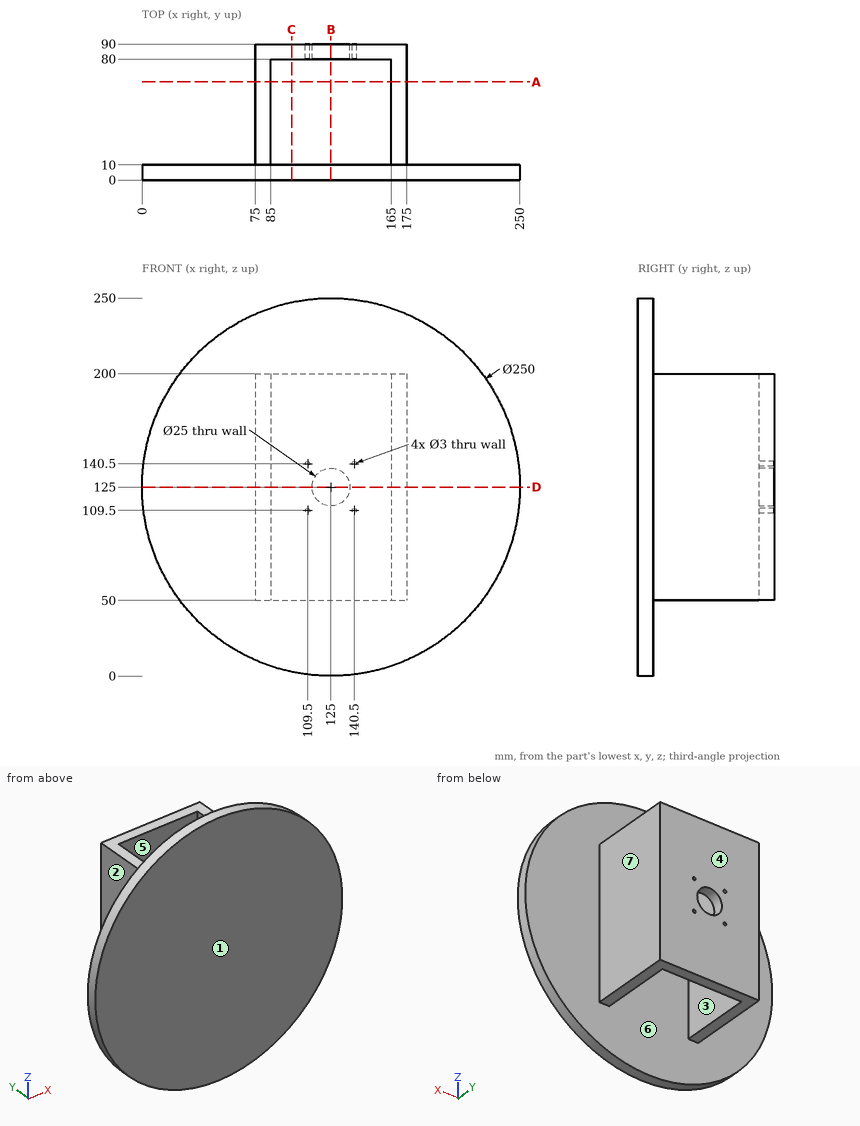
Study the drawing (mm; zero at the part's minimum x, y, z) and answer. A direction names the side the tool comes from. Coordinates: 2 decimals unless noted, no trailing zeros. Loops run counter-clockwise (first coordinate to the right, second up) from the corner with the lowest first, then second, coordinate; pieces in that order, holes last. Notation, with made-up numbers: (38, -18) -> (81, -18) arc R27 ccw to (81, -1) -> close; hole circle Ø4 at (-29.5, 7). An arc over 180 degrees is marked (long way). Answer as CSV lines item,"result".
1) For the marked faces 1, 2 and 3, determine the directions among +Z, -Z, +X, -X, +Y, -Y from which every point of the face is accessible in a straight line to the end or side of a thin tool.
A:
face 1,"+Z, -Z, +X, -X, -Y"
face 2,"+Z, -Z, -X, +Y"
face 3,"+Z, -Z"
2) The part is cut by section D-D (z = 125). Give the vertices of the cut face in (x, y), and give its area (3 significant figures).
A:
outline,"(0, 0) -> (250, 0) -> (250, 10) -> (175, 10) -> (175, 90) -> (137.5, 90) -> (137.5, 80) -> (165, 80) -> (165, 10) -> (85, 10) -> (85, 80) -> (112.5, 80) -> (112.5, 90) -> (75, 90) -> (75, 10) -> (0, 10) -> close"
area,"4,650 mm²"
3) Flat-ended cylindrical pins translate along their axes: pin 1 (24 mm diameter, centred on y = 47.5, z = 129, fed in from +X); pin 2 (2 mm diameter, centred on y = 19.5, z = 174.5, fed in from -X); pin 3 (2.5 mm diameter, centred on x = 140.5, z = 140.5, fed in from +Y); pin 4 (24 mm diameter, centred on x = 112.5, y = 57.5, fed in from -Z). Find the tip coordinate at first contact, or state that the pin passes through.
A:
pin 1,"stops at x = 175"
pin 2,"stops at x = 75"
pin 3,"stops at y = 10"
pin 4,"passes through"
4) Straight lines are drawn through the part: probe 1 along X at (y, z) = (85, 140.5); probe 2 along Z at (x, y) = (140.5, 84.25); probe 3 along X at (y, z) = (48, 145). For each, find the intervals that lie inside material, in ascending order.
A:
probe 1,"x = 75 to 108, 111 to 139, 142 to 175"
probe 2,"z = 50 to 108, 111 to 139, 142 to 200"
probe 3,"x = 75 to 85, 165 to 175"
5) The part is cut by section A-A (y = 65). Give the vertices of the cut face in (x, z).
A:
outline,"(75, 50) -> (85, 50) -> (85, 200) -> (75, 200) -> close; (165, 50) -> (175, 50) -> (175, 200) -> (165, 200) -> close"
6) The part is cut by section C-C (x = 99). Give the vertices of the cut face in (y, z).
A:
outline,"(0, 2.73) -> (10, 2.73) -> (10, 247.27) -> (0, 247.27) -> close; (80, 50) -> (90, 50) -> (90, 200) -> (80, 200) -> close"
7) The part is cut by section B-B (x = 125). Give the vertices of the cut face in (y, z).
A:
outline,"(0, 0) -> (10, 0) -> (10, 250) -> (0, 250) -> close; (80, 50) -> (90, 50) -> (90, 112.5) -> (80, 112.5) -> close; (80, 137.5) -> (90, 137.5) -> (90, 200) -> (80, 200) -> close"
8) For a pull along X with two mould halves and no side action, classify the marked faces 4, 5, 6 and 7 as released by +X, released by -X, zero draft, split by the parting line, or undercut.
A:
face 4,"zero draft"
face 5,"undercut"
face 6,"undercut"
face 7,"released by +X"
